Design review of the part shown in the three views and the two pictorial views. Dimensions are in mm from the part's minimum x, y and z. Round coordinates to 2 decimals unless told otherwise and drop trailing zeros. Loops run counter-clockwise (first coordinate to the right, second up) from the corner with the lowest first, then second, coordinate; pieces in that order, holes last. Notation, with made-up numbers: (78.5, 54) -> (106.5, 54) arc R13 ccw to (106.5, 69) -> close; hole circle Ø3 at (19, -39). An arc over 180 degrees is marked (long way). One line per question, with ' | ' between items. Start each with the question number.
1. Consider section D-D (x = 15.5). Write out the cut boundary in (y, z).
2. Consider section B-B (y = 6.5). Write out the cut boundary in (x, z), and give its area (3 significant figures).
3. Wall thickness on line 1 along Y through (x, z) = (33, 3); line 2 along Y through (x, z) = (33, 5.25); line 3 along Z through (x, y) = (6, 4.5): over which ranges is each line inside the solid? List them lowest first.
4. Consider section C-C (z = 2). Write out the cut boundary in (x, y), and give its area (3 significant figures).
5. For pin 1 Ø1 at (x, z) = (31.5, 6.5) entering from -Y; pin 2 Ø1.5 at (y, z) = (21.5, 6) entering from -X; pin 3 Ø7.5 at (x, y) = (18.5, 7.5) entering from +Z, all flat-tipped, find the tip position at first contact; note any pin that passes through.
6. Draft analysis for pull direction X (two halves, no side actions). For the marked faces 1, 2, 3 and 4, state which applies: pulls with the +X half, pulls with the -X half, needs draft (parallel to the pull), parting line crosses it, or undercut.
7. Consider section A-A (x = 33). Write out the cut boundary in (y, z), and give its area (3 significant figures).
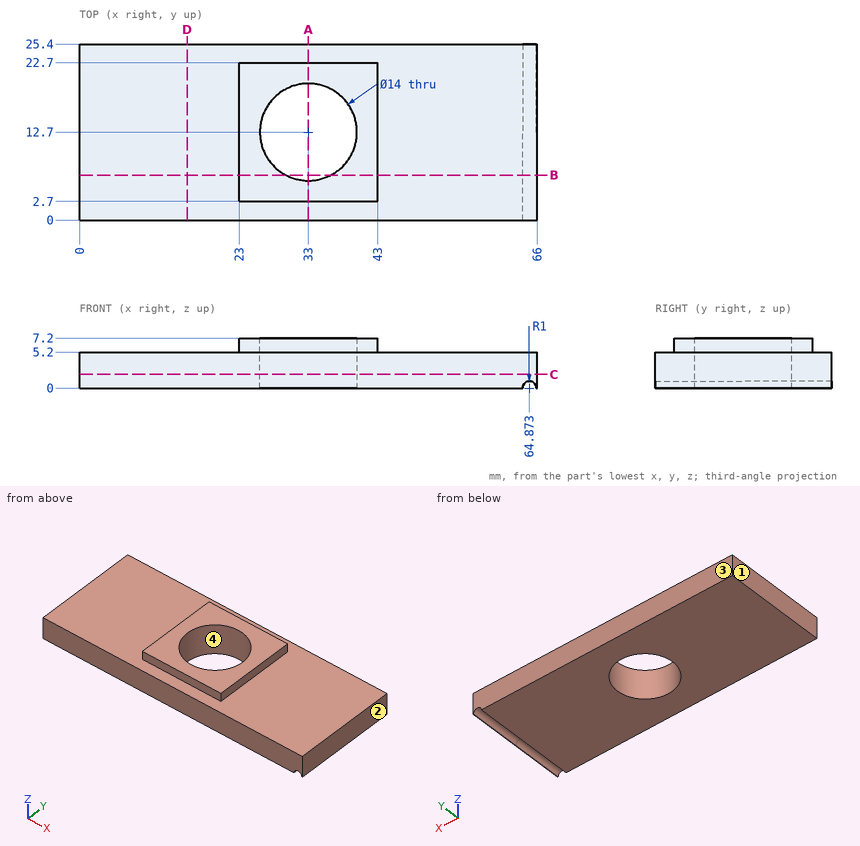
Answer block:
1) outline: (0, 0) -> (25.4, 0) -> (25.4, 5.2) -> (0, 5.2) -> close
2) outline: (0, 0) -> (29.75, 0) -> (29.75, 7.2) -> (23, 7.2) -> (23, 5.2) -> (0, 5.2) -> close; (36.25, 0) -> (63.87, 0) arc R1 cw to (65.87, 0) -> (66, 0) -> (66, 5.2) -> (43, 5.2) -> (43, 7.2) -> (36.25, 7.2) -> close | area: 335 mm2
3) line 1: y = 0 to 5.7, 19.7 to 25.4 | line 2: y = 2.7 to 5.7, 19.7 to 22.7 | line 3: z = 0 to 5.2
4) outline: (0, 0) -> (66, 0) -> (66, 25.4) -> (0, 25.4) -> close; hole circle Ø14 at (33, 12.7) | area: 1,520 mm2
5) pin 1: stops at y = 2.7 | pin 2: stops at x = 23 | pin 3: stops at z = 5.2
6) face 1: pulls with the -X half | face 2: pulls with the +X half | face 3: needs draft | face 4: undercut
7) outline: (0, 0) -> (5.7, 0) -> (5.7, 7.2) -> (2.7, 7.2) -> (2.7, 5.2) -> (0, 5.2) -> close; (19.7, 0) -> (25.4, 0) -> (25.4, 5.2) -> (22.7, 5.2) -> (22.7, 7.2) -> (19.7, 7.2) -> close | area: 71.3 mm2
